Here's how the part is built. I have some questions about the finished solid (model axes, mm). Face numbers are marked on the shaded views. A direction names the side the tool comes from. Round coordinates to 2 decimals unless told otherwise and drop trailing zeros. Write each loop counter-clockwise with the first axis right and the second up, starting at its lowest first coordinate (ties: lowest second). Pieces come first, ordered by that corner, then holes. Notation, with made-up numbers: (-3, -39.5) - (40, -39.5) arc R24 cw to (40, -5.5) - close; hole circle Ø6 at (32, -29.75). An arc over 180 degrees is marked (long way). Return JSON: item names as keys, results as strings. Group by question number.
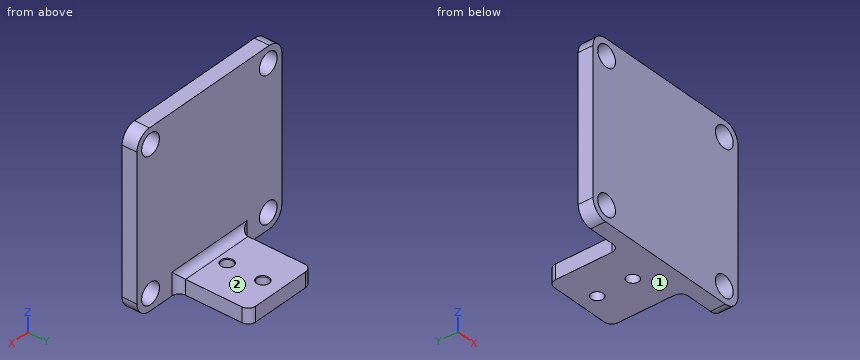
```python
from build123d import *

# Parameters (mm, degrees)
SKETCH1_W                         = 58
SKETCH1_H                         = 58
SKETCH1_R                         = 3.55
BOSS_EXTRUDE1_DEPTH               = 5
FILLET1_R                         = 5
BOSS_EXTRUDE2_START               = -29
SKETCH5_W                         = 25
SKETCH5_H                         = 24
BOSS_EXTRUDE2_DEPTH               = 5
F_4_0_4_DIAMETER_HOLE1_AT_2_COUNT = 2
F_4_0_4_DIAMETER_HOLE1_AT_2_PITCH = 12
FILLET2_R                         = 2.5


with BuildPart() as part:
    # Sketch1 → Boss-Extrude1 (new body)
    with BuildSketch(Plane(origin=(0, 0, 0), x_dir=(1, 0, 0), z_dir=(0, 1, 0))):
        Rectangle(SKETCH1_W, SKETCH1_H)
        with Locations(Location((-23.57, 23.57, 0), (0, 0, 270))):
            Circle(SKETCH1_R, mode=Mode.SUBTRACT)
        with Locations(Location((23.57, 23.57, 0), (0, 0, 270))):
            Circle(SKETCH1_R, mode=Mode.SUBTRACT)
        with Locations(Location((23.57, -23.57, 0), (0, 0, 270))):
            Circle(SKETCH1_R, mode=Mode.SUBTRACT)
        with Locations(Location((-23.57, -23.57, 0), (0, 0, 270))):
            Circle(SKETCH1_R, mode=Mode.SUBTRACT)
    extrude(amount=BOSS_EXTRUDE1_DEPTH)

    # Fillet1
    fillet1_edges = [part.edges().sort_by_distance(p)[0] for p in [
        (29, 2.5, 29),
        (-29, 2.5, 29),
        (-29, 2.5, -29),
        (29, 2.5, -29),
    ]]
    fillet(fillet1_edges, radius=FILLET1_R)

    # Sketch5 → Boss-Extrude2 (add)
    with BuildSketch(Plane.XY.offset(BOSS_EXTRUDE2_START)):
        with Locations((0, 17)):
            Rectangle(SKETCH5_W, SKETCH5_H)
    extrude(amount=BOSS_EXTRUDE2_DEPTH)

    # Sketch7 → Ø4.0 (4) Diameter Hole1 (revolve, cut)
    with BuildSketch(Plane(origin=(0, 11, -24), x_dir=(0, -1, 0), z_dir=(1, 0, 0))):
        Polygon((0, 0), (0, 5), (2, 5), (2, 0.301776695), (2.125, 0), align=None)
    f_4_0_4_diameter_hole1 = revolve(axis=Axis((0, 11, -17.65), (0, 0, -1)), mode=Mode.SUBTRACT)

    # Ø4.0 (4) Diameter Hole1 at 2: Ø4.0 (4) Diameter Hole1 ×2
    with Locations(*[(0, i * F_4_0_4_DIAMETER_HOLE1_AT_2_PITCH, 0) for i in range(1, F_4_0_4_DIAMETER_HOLE1_AT_2_COUNT)]):
        add(f_4_0_4_diameter_hole1, mode=Mode.SUBTRACT)

    # Fillet2
    fillet2_edges = [part.edges().sort_by_distance(p)[0] for p in [
        (-12.5, 5, -26.5),
        (12.5, 5, -26.5),
        (12.5, 29, -26.5),
        (-12.5, 29, -26.5),
        (0, 5, -24),
    ]]
    fillet(fillet2_edges, radius=FILLET2_R)


solid = part.part
```
1) For the marked faces 1 and 2, which set-ups out of +Z, -Z, +X, -X, +Y, -Y let a thin tool reach every point of the face, with its end or its side?
2) Will these pins go through, and if not, where does the flat tip stop? pin 1 Ø12 at (x, z) = (11.5, 12.5) entering from +Y; pin 2 Ø2.5 at (x, y) = (0, 11) entering from +Z; pin 3 Ø4 at (y, z) = (14.5, -27) entering from -X; pin 4 Ø5 at (x, y) = (-11.5, 24.5) entering from +Z.
3) Imagine slicing it at A-A (y = 23). Please give me the cut outline in (x, z) (3 decimals), plus the area to 3 significant figures.
4) Imagine slicing it at B-B (x = 3). Please give me the cut outline in (y, z).
5) I need wall thicknesses on line 1 along X through (y, z) = (1.35, -23.57); line 2 along Y through (x, z) = (0, -27.2); line 3 along X through (y, z) = (2.25, 23). Which ranges of each line are inside material? Lowest first, please.
6) Imagine slicing it at C-C (z = -13). Please give me the cut outline in (x, y).
Results found:
{
 "1": {"face 1": "-Z, +X, -X, +Y, -Y", "face 2": "+Z, +X, -X, +Y"},
 "2": {"pin 1": "stops at y = 5", "pin 2": "passes through", "pin 3": "stops at x = -12.5", "pin 4": "stops at z = -24"},
 "3": {"outline": "(-12.5, -29) - (-2, -29) - (-2, -24.302) - (-2.125, -24) - (-12.5, -24) - close; (2, -29) - (12.5, -29) - (12.5, -24) - (2.125, -24) - (2, -24.302) - close", "area": "105 mm²"},
 "4": {"outline": "(0, -29) - (29, -29) - (29, -24) - (7.5, -24) arc R2.5 cw to (5, -21.5) - (5, 29) - (0, 29) - close"},
 "5": {"line 1": "x = -29 to -27.12, -20.02 to 20.02, 27.12 to 29", "line 2": "y = 0 to 9, 13 to 21, 25 to 29", "line 3": "x = -29 to -27.07, -20.07 to 20.07, 27.07 to 29"},
 "6": {"outline": "(-29, 0) - (29, 0) - (29, 5) - (-29, 5) - close"}
}
